from build123d import *

# Parameters (mm, degrees)
F0_R     = 17.5895
F1_DEPTH = 3.175


with BuildPart() as f1:
    # F0 (on Top) → F1 (new body)
    with BuildSketch(Plane.XY):
        Circle(F0_R)
        with BuildLine():
            Line((-4.2164, 5.4102), (5.4102, 5.4102))
            ThreePointArc((5.4102, 5.4102), (6.0071, 4.8133), (5.4102, 4.2164))
            Line((5.4102, 4.2164), (5.4102, -5.4102))
            ThreePointArc((5.4102, -5.4102), (4.8133, -6.0071), (4.2164, -5.4102))
            Line((4.2164, -5.4102), (-5.4102, -5.4102))
            ThreePointArc((-5.4102, -5.4102), (-6.0071, -4.8133), (-5.4102, -4.2164))
            Line((-5.4102, -4.2164), (-5.4102, 5.4102))
            ThreePointArc((-5.4102, 5.4102), (-4.8133, 6.0071), (-4.2164, 5.4102))
        make_face(mode=Mode.SUBTRACT)
    extrude(amount=F1_DEPTH)


solid = f1.part
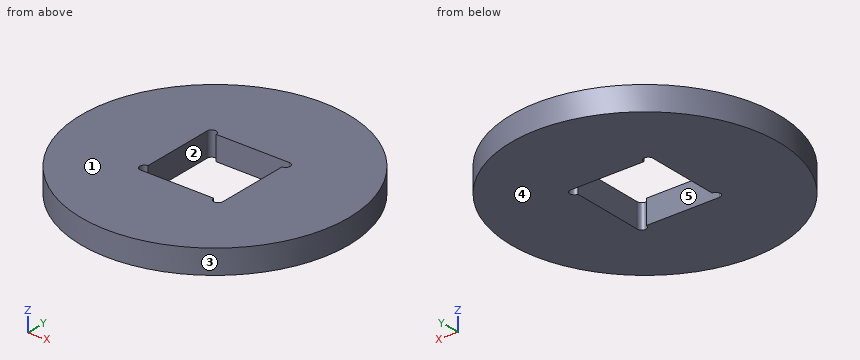
The listing builds one solid part. Answer for the finished solid, in the listing's coordinates (mm). Face numbers are marked on the shaded views. A direction names the side the tool comes from. Coordinates: 2 decimals unless noted, no trailing zeros. Loops run counter-clockwise (first coordinate to the right, second up) from the corner with the lowest first, then second, coordinate; pieces in that order, holes last. Notation, with made-up numbers: (11, 48.5) -> (45, 48.5) arc R13 ccw to (45, 59.5) -> close; hole circle Ø10 at (87.25, 1). An arc over 180 degrees is marked (long way). Write item = value, one per line. Start each with the question number.
1) A cutting plane is placed at D-D (y = 15). Give the vertices of the cut face in (x, z) (3 decimals).
2) Straight lines are drawn through the part: line 1 (Y direction, x = -0.5, z = 1.3); line 2 (Y direction, x = -3, z = 2.2); line 3 (X direction, y = -2.5, z = 0.25). For each, find the intervals that lie inside material, in ascending order. Write a range as from..to.
3) A cutting plane is placed at A-A (x = 0). Give the vertices of the cut face in (y, z) (1 decimal).
4) The mould has two halves that part along Y. Classify the marked faces 3, 4 and 5: released by +Y, released by -Y, zero draft, split by the parting line, or undercut.
5) Given pin 1 Ø1.6 at (x, z) = (0.5, 2.5) entering from +Y; pin 2 Ø1.6 at (y, z) = (1, 1.5) entering from -X; pin 3 Ø1.6 at (x, z) = (-1.5, 2.5) entering from -Y, each flat-ended and moving along its own axis, determine where each tip first touches the part or whether it passes through.
6) A cutting plane is placed at C-C (z = 0.7). Give the vertices of the cut face in (x, y).
7) A tool of negligible diameter and unlimited length cuts with its end or side. For the marked faces 1 and 2, from which of +Z, -Z, +X, -X, +Y, -Y can it reach the whole face along a straight path? Write none if from no direction.
Responses:
q1.outline = (-9.186, 0) -> (9.186, 0) -> (9.186, 3.175) -> (-9.186, 3.175) -> close
q2.line_1 = -17.58..-5.41, 5.41..17.58
q2.line_2 = -17.33..-5.41, 5.41..17.33
q2.line_3 = -17.41..-5.41, 5.41..17.41
q3.outline = (-17.6, 0) -> (-5.4, 0) -> (-5.4, 3.2) -> (-17.6, 3.2) -> close; (5.4, 0) -> (17.6, 0) -> (17.6, 3.2) -> (5.4, 3.2) -> close
q4.face_3 = split by the parting line
q4.face_4 = zero draft
q4.face_5 = undercut
q5.pin_1 = 17.59
q5.pin_2 = -17.59
q5.pin_3 = -17.58
q6.outline = circle Ø35.18 at (0, 0); hole (-5.41, -5.41) -> (4.22, -5.41) arc R0.6 ccw to (5.41, -5.41) -> (5.41, 4.22) arc R0.6 ccw to (5.41, 5.41) -> (-4.22, 5.41) arc R0.6 ccw to (-5.41, 5.41) -> (-5.41, -4.22) arc R0.6 ccw to start
q7.face_1 = +Z, +X, -X, +Y, -Y
q7.face_2 = +Z, -Z
